from build123d import *

# Parameters (mm, degrees)
SKETCH1_W               = 76.2
SKETCH1_H               = 19.05
BASE_FLANGE1_DEPTH      = 3.175
EDGE_FLANGE1_DEPTH      = 76.2
EDGE_FLANGE2_DEPTH      = 76.2
F_1_4_CLEARANCE_HOLE1_D = 6.7564
SKETCH17_W              = 165.1
SKETCH17_H              = 25.4
BOSS_EXTRUDE1_DEPTH     = 3.175
F_1_4_CLEARANCE_HOLE3_D = 6.7564
FILLET1_R               = 6.35


# Sheet-metal steps are written as plain solids
with BuildPart() as part:
    # Sketch1 → Base-Flange1 (new body)
    with BuildSketch(Plane(origin=(0, 0, 0), x_dir=(1, 0, 0), z_dir=(0, 1, 0))):
        with Locations((0, -9.525)):
            Rectangle(SKETCH1_W, SKETCH1_H)
    extrude(amount=-BASE_FLANGE1_DEPTH)

    # Edge-Flange1 section (across the edge) → Edge-Flange1 (add)
    with BuildSketch(Plane(origin=(38.1, -3.175, 20.883087105), x_dir=(0, -0.5000000000000041, -0.8660254037844364), z_dir=(-1, 0, 0))):
        with BuildLine():
            Line((-3.175, 1.833087105), (-3.175, 36.266912895))
            Line((-3.175, 36.266912895), (0, 36.266912895))
            Line((0, 36.266912895), (0, 1.833087105))
            ThreePointArc((0, 1.833087105), (0.425369343, 0.245587105), (1.5875, -0.916543552))
            Line((1.5875, -0.916543552), (0, -3.666174209))
            ThreePointArc((0, -3.666174209), (-2.324261314, -1.341912895), (-3.175, 1.833087105))
        make_face()
    extrude(amount=EDGE_FLANGE1_DEPTH)

    # Edge-Flange2 section (across the edge) → Edge-Flange2 (add)
    with BuildSketch(Plane(origin=(-38.1, -33.732329198, 42.191543552), x_dir=(0, 0.866025403784438, 0.5000000000000012), z_dir=(1, 0, 0))):
        with BuildLine():
            Line((-3.175, 0.850738686), (-3.175, 49.949261314))
            Line((-3.175, 49.949261314), (0, 49.949261314))
            Line((0, 49.949261314), (0, 0.850738686))
            ThreePointArc((0, 0.850738686), (0.108185502, 0.028988218), (0.425369343, -0.736761314))
            Line((0.425369343, -0.736761314), (-2.324261314, -2.324261314))
            ThreePointArc((-2.324261314, -2.324261314), (-2.958628997, -0.79276225), (-3.175, 0.850738686))
        make_face()
    extrude(amount=EDGE_FLANGE2_DEPTH)

    # 1/4 Clearance Hole1 (through all)
    with Locations(Plane(origin=(0, 0, 0), x_dir=(1, 0, 0), z_dir=(0, 1, 0))):
        with Locations((-31.75, -9.525), (31.75, -9.525)):
            Hole(F_1_4_CLEARANCE_HOLE1_D / 2)

    # Sketch17 → Boss-Extrude1 (add)
    with BuildSketch(Plane(origin=(0, -7.029772628, -4.058641119), x_dir=(1, 0, 0), z_dir=(0, 0.866025403784438, 0.5000000000000012))):
        with Locations((0, -90.654374454)):
            Rectangle(SKETCH17_W, SKETCH17_H)
    extrude(amount=-BOSS_EXTRUDE1_DEPTH)

    # 1/4 Clearance Hole3 (through all)
    with Locations(Plane(origin=(0, -7.029772628, -4.058641119), x_dir=(1, 0, 0), z_dir=(0, 0.866025403784438, 0.5000000000000012))):
        with Locations((76.2, -90.654374454), (-76.2, -90.654374454)):
            Hole(F_1_4_CLEARANCE_HOLE3_D / 2)

    # Fillet1
    fillet1_edges = [part.edges().sort_by_distance(p)[0] for p in [
        (82.55, -60.081775184, 84.655122751),
        (-82.55, -47.381775184, 62.658077494),
        (82.55, -47.381775184, 62.658077494),
        (-82.55, -60.081775184, 84.655122751),
        (-38.1, -47.381775184, 62.658077494),
        (38.1, -47.381775184, 62.658077494),
        (-38.1, -1.5875, 0),
        (38.1, -1.5875, 0),
    ]]
    fillet(fillet1_edges, radius=FILLET1_R)


solid = part.part
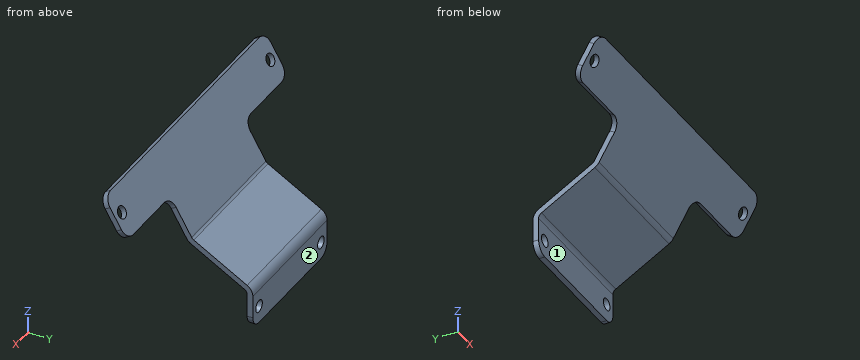
The model under review builds one solid part; all positions refer to its coordinate system, in mm. Face numbers are marked on the shaded views. A direction names the side the tool comes from. Give positions to 0.01 mm unless a question says otherwise; leave off trailing zeros. Order: outer loops, then holes, each group sorted by start corner. A loop starts at its lowest first (then second) coordinate and runs counter-clockwise, first axis right, second up. Notation, with made-up numbers: M 55,77.5 L 62,77.5 A35 cw 62,111.5 Z; hole C 76,55 d1. An arc over 180 degrees is marked long. One line per question, with ' | ' between items. Start each with the question number.
1) Consider section B-B, the plane z = 15.5. Give the boundary of the cut face in (x, y) (3 decimals), then the cut area to 3 significant figures.
2) For the marked faces 1 and 2, list the 3-axis set-ups (+Z, -Z, +X, -X, +Y, -Y) from which the entire face can be reached by the end or side of a thin tool; tool diameter is ignored.
3) Consider section C-C, the plane y = -30.5. Give the boundary of the cut face in (x, z).
4) Clearance check with flat-ended pins moving along their axes: P1, Ø21, axis at x = -15, z = 9, coming from the -Y side; P2, Ø6, axis at y = -36.5, z = 51, coming from the +X side; P3, Ø6, axis at x = -15, y = -27, coming from the -Z side. State where each tip first meets the part, or that it passes through.
5) Wall thickness on L1, parallel to Y at x = -33, z = 4.5 (3 decimals); L2, parallel to Z at x = -31.75, y = -2.5; L3, parallel to Y at x = -20, z = 29: over which ranges is each line inside the solid? List them lowest first. Write a range as from..to.
Found:
1) outline: M -38.1,-3.175 L 38.1,-3.175 L 38.1,0 L -38.1,0 Z | area: 242 mm²
2) face 1: -Z, +X, -X, -Y | face 2: +Z, -Z, +X, -X, +Y
3) outline: M -38.1,36.66 L 38.1,36.66 L 38.1,40.33 L -38.1,40.33 Z
4) P1: stops at y = -3.21 | P2: stops at x = 38.1 | P3: stops at z = 32.91
5) L1: y = -3.175..0 | L2: z = 0..6.15, 12.9..24.1 | L3: y = -17.23..-10.88
